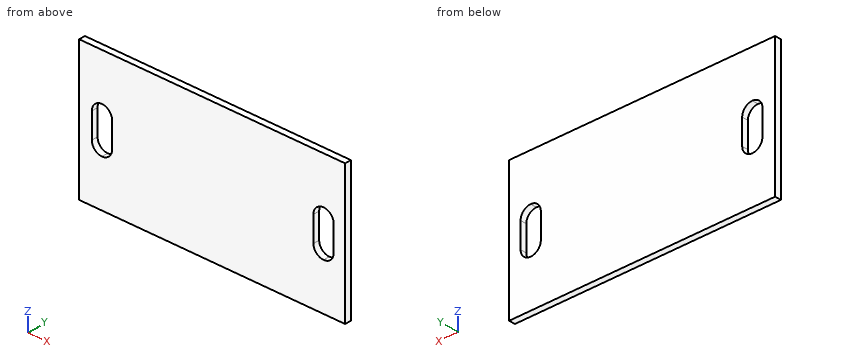
from build123d import *

# Parameters (mm, degrees)
F0_W     = 210
F0_H     = 110
F0_W_2   = 16
F0_H_2   = 36
F1_DEPTH = 5
F2_R     = 7.99999


# Not quite as in the source:
# - a fillet or chamfer is up to 0.001 mm smaller than in the source, because OpenCascade refuses the exact size
# - a feature names something its author has since deleted; it is built from what else it names


with BuildPart() as f1:
    # F0 (on Front) → F1 (new body)
    with BuildSketch(Plane.XZ):
        Rectangle(F0_W, F0_H)
        with Locations((-87, 0)):
            Rectangle(F0_W_2, F0_H_2, mode=Mode.SUBTRACT)
        with Locations((88, 0)):
            Rectangle(F0_W_2, F0_H_2, mode=Mode.SUBTRACT)
    extrude(amount=F1_DEPTH)

    # F2 (radius 8 in the source; OpenCascade refuses exactly that, so slightly less here)
    f2_edges = [f1.edges().sort_by_distance(p)[0] for p in [
        (-95, -2.5, 18),
        (-79, -2.5, 18),
        (-95, -2.5, -18),
        (-79, -2.5, -18),
        (80, -2.5, 18),
        (96, -2.5, 18),
        (96, -2.5, -18),
        (80, -2.5, -18),
    ]]
    fillet(f2_edges, radius=F2_R)


solid = f1.part
Here's how the part is built. I have some questions about the finished solid (model axes, mm). Coordinates: 2 decimals unless noted, no trailing zeros. Order: outer loops, then holes, each group sorted by start corner. A loop starts at its lowest first (then second) coordinate and runs counter-clockwise, first axis right, second up. Notation, with made-up numbers: M 36,49 L 85,49 A18 ccw 85,66 Z; hole C 69,28 d9. An arc over 180 degrees is marked long. Answer as CSV lines item,"result".
Item 1: Imagine slicing it at B-B on x = 91. Write out the boundary of the cut face in (y, z), plus the area to 3 significant figures.
Results found:
outline,"M -5,-55 L 0,-55 L 0,-17.42 L -5,-17.42 Z; M -5,17.42 L 0,17.42 L 0,55 L -5,55 Z"
area,"376 mm2"
Item 2: If I drill on line 1 (X direction, y = -2.2, z = -6); line 2 (X direction, y = -3.9, z = -13.5); line 3 (Z direction, x = 90, y = -0.65), over which ranges is the centre line in solid material (lowest first)?
Results found:
line 1,"-105 to -95, -79 to 80, 96 to 105"
line 2,"-105 to -94.19, -79.81 to 80.81, 95.19 to 105"
line 3,"-55 to -17.75, 17.75 to 55"
Item 3: Imagine slicing it at A-A on y = -2.3. Give the number of separate pieces and of enclosed holes in the cut face, plus the area to 3 significant figures.
Results found:
separate pieces,"1"
enclosed holes,"2"
area,"22,100 mm2"
